Autodesk Inventor part; units mm, degrees
ref_plane "YZ Plane" through (0, 0, 0) normal (1, 0, 0) x (0, 1, 0)
ref_plane "XZ Plane" through (0, 0, 0) normal (0, 1, 0) x (-1, 0, 0)
ref_plane "XY Plane" through (0, 0, 0) normal (0, 0, 1) x (1, 0, 0)
sketch "Sketch1" plane through (0, 0, 0) normal (0, 1, 0) x (-1, 0, 0)
  line L0 (-4, 0) -> (-44, 0)
  line L1 (-48, -4) -> (-48, -61)
  line L2 (-44, -65) -> (-4, -65)
  line L3 (0, -61) -> (0, -4)
  arc A0 (0, -4) -> (-4, 0) centre (-4, -4) ccw
  arc A1 (-4, -65) -> (0, -61) centre (-4, -61) ccw
  arc A2 (-48, -61) -> (-44, -65) centre (-44, -61) ccw
  arc A3 (-44, 0) -> (-48, -4) centre (-44, -4) ccw
  line L4 (-48, -65) -> (-42, -65)
  line L5 (-48, -59) -> (-48, -65)
  line L6 (0, 0) -> (-6, 0)
  line L7 (0, -6) -> (0, 0)
  circle A4 centre (-6, -6) radius 1
  circle A5 centre (-42, -59) radius 1
  line L8 (-14.6534, -26.5) -> (-14.6534, -38.5)
  line L9 (-14.6534, -38.5) -> (-9.6534, -38.5)
  line L10 (-9.6534, -38.5) -> (-9.6534, -26.5)
  line L11 (-9.6534, -26.5) -> (-14.6534, -26.5)
  line L12 (-9.6534, -26.5) -> (-9.6534, -19.5)
  line L13 (-9.6534, -19.5) -> (-35.6534, -19.5)
  line L14 (-35.6534, -19.5) -> (-35.6534, -45.5)
  line L15 (-35.6534, -45.5) -> (-9.6534, -45.5)
  line L16 (-9.6534, -45.5) -> (-9.6534, -19.5)
  point P0 (-48, 0)
  point P1 (0, -65)
  dimension "d0" = 48
  dimension "d1" = 65
  dimension "d3" = 4
extrude "Extrusion1" add sketch "Sketch1" along normal blind 3 contours A0 L3 A1 L2 A2 L1 A3 L0
sketch "Sketch3" plane through (0, 3, 0) normal (0, 1, 0) x (1, 0, 0)
  line L0 (9.6534, 19.5) -> (9.6534, 45.5)
  line L1 (9.6534, 45.5) -> (9.6534, 38.5)
  line L2 (9.6534, 38.5) -> (14.6534, 38.5)
  line L3 (14.6534, 38.5) -> (14.6534, 26.5)
  line L4 (14.6534, 26.5) -> (9.6534, 26.5)
  line L5 (9.6534, 26.5) -> (9.6534, 38.5)
  line L6 (35.6534, 19.5) -> (9.6534, 19.5)
  line L7 (9.6534, 45.5) -> (35.6534, 45.5)
  line L8 (35.6534, 45.5) -> (35.6534, 19.5)
  line L9 (35.6534, 19.5) -> (9.6534, 19.5)
  line L10 (9.6534, 19.5) -> (9.6534, 45.5)
  line L11 (9.6534, 19.5) -> (11.6534, 19.5)
  line L12 (9.6534, 21.5) -> (9.6534, 19.5)
  circle A0 centre (11.6534, 21.5) radius 1.5
  line L13 (35.6534, 45.5) -> (35.6534, 19.5)
  line L14 (9.6534, 45.5) -> (35.6534, 45.5)
  circle A1 centre (11.6534, 43.5) radius 1.5
  circle A2 centre (33.5528, 21.5) radius 1.5
  circle A3 centre (33.5528, 43.5) radius 1.5
  point P0 (0, 0)
  dimension "d20" = 5
  dimension "d21" = 12
extrude "Extrusion2" add sketch "Sketch3" against normal blind 2 contours L0 L4 L3 L2 L7 L8 L6
properties part number "Tampa"
The model under review builds one solid part; all positions refer to its coordinate system, in mm. A direction names the side the tool comes from. Round coordinates to 2 decimals unless told otherwise and drop trailing zeros. Loops run counter-clockwise (first coordinate to the right, second up) from the corner with the lowest first, then second, coordinate; pieces in that order, holes last. Notation, with made-up numbers: M 38.25,58 L 86.25,58 A27 cw 86.25,96 Z; hole C 27.25,10.25 d7. An arc over 180 degrees is marked long. Answer as a JSON object with one key per item and string values.
(1) Clearance check with flat-ended pins moving along their axes: P1, Ø1.6, axis at y = 1.5, z = -32.5, coming from the -X side; P2, Ø1.5, axis at x = 16, z = -34.5, coming from the -Y side. State where each tip first meets the part, or that it passes through.
Resolved:
{"P1": "x = 0", "P2": "y = 1"}
(2) Take a section at A-A on z = -21.5. Give the boundary of the cut face in (x, y), and give its area (3 significant figures).
Resolved:
{"outline": "M 0,0 L 9.65,0 L 9.65,1 L 10.15,1 L 10.15,3 L 0,3 Z; M 13.15,1 L 32.05,1 L 32.05,3 L 13.15,3 Z; M 35.05,1 L 35.65,1 L 35.65,0 L 48,0 L 48,3 L 35.05,3 Z", "area": "106 mm²"}
(3) Take a section at D-D on y = 2.35. Give the boundary of the cut face in (x, z).
Resolved:
{"outline": "M 0,-61 A4 ccw 4,-65 L 44,-65 A4 ccw 48,-61 L 48,-4 A4 ccw 44,0 L 4,0 A4 ccw 0,-4 Z; hole C 6,-6 d2; hole M 9.65,-38.5 L 14.65,-38.5 L 14.65,-26.5 L 9.65,-26.5 Z; hole C 11.65,-43.5 d3; hole C 11.65,-21.5 d3; hole C 33.55,-43.5 d3; hole C 33.55,-21.5 d3; hole C 42,-59 d2"}
(4) To check wall thickness, follow line 1 along Z through (x, y) = (17, 0.75); line 2 along X through (y, z) = (2.2, -28.5); line 3 along X through (y, z) = (1.95, -21.5). State the ranges of each line that lie inside material, in increasing order.
Resolved:
{"line 1": "-65 to -45.5, -19.5 to 0", "line 2": "0 to 9.65, 14.65 to 48", "line 3": "0 to 10.15, 13.15 to 32.05, 35.05 to 48"}
(5) Draft analysis for pull direction Z (two halves, no side actions). For faces 1 (the flat face through (24, 3, -32)), 2 (the cylindrical face through (46.859, 1.479, -1.203)), 3 (the cylindrical face through (12.46, 2.014, -22.765)), state which applies: released by +Z, released by -Z, zero draft, split by the parting line, or undercut.
Resolved:
{"face 1": "zero draft", "face 2": "released by +Z", "face 3": "undercut"}
(6) Take a section at C-C on z = -35.5. Give the boundary of the cut face in (x, y).
Resolved:
{"outline": "M 0,0 L 9.65,0 L 9.65,3 L 0,3 Z; M 14.65,1 L 35.65,1 L 35.65,0 L 48,0 L 48,3 L 14.65,3 Z"}
(7) Tool access review of faces 4 (the flat face through (12, 2, -38.5)), 5 (the flat face through (9.653, 1, -33)), 6 (the flat face through (24, 1, 0)): name each direction out of +Z, -Z, +X, -X, +Y, -Y from which nothing blocks a thin tool from reaching the whole face with its end or side.
Resolved:
{"face 4": "+Y, -Y", "face 5": "-Y", "face 6": "+Z, +X, -X, +Y, -Y"}
(8) Take a section at B-B on x = 42. Give the boundary of the cut face in (y, z), and give its area (3 significant figures).
Resolved:
{"outline": "M 0,-65 L 3,-65 L 3,-60 L 0,-60 Z; M 0,-58 L 3,-58 L 3,0 L 0,0 Z", "area": "189 mm²"}
